Can you work these out from the drawing? Everything is in mm from the part's minimum corner. Give positions to 0.01 mm unless a question says otherwise; leave off trailing zeros. Write each loop counter-clockwise with the first axis right and the second up, starting at its lowest first coordinate (ties: lowest second). Pieces come first, ordered by that corner, then holes. Notation, with made-up numbers: M 89.5,-22.75 L 146.5,-22.75 A27 cw 146.5,-0.75 Z; hole C 66,83 d9. An arc over 180 degrees is marked long. One line per item, written item: value.
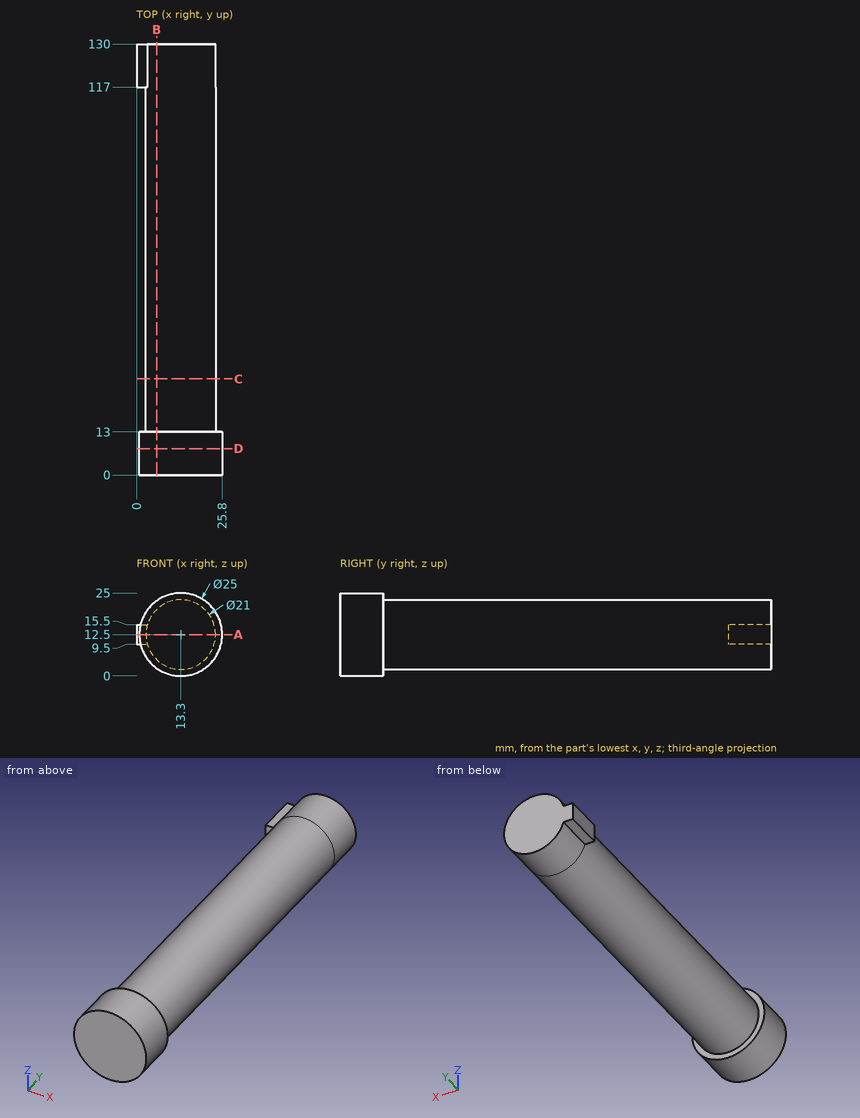
1) If we section it at D-D, the plane y = 8: Write out the boundary of the cut face in (x, z), then the cut area to 3 significant figures.
Outcome:
outline: C 13.3,12.5 d25
area: 491 mm^2
2) If we section it at B-B, the plane x = 6: Write out the boundary of the cut face in (y, z), then the cut area to 3 significant figures.
Outcome:
outline: M 0,2.35 L 13,2.35 L 13,4.95 L 130,4.95 L 130,20.05 L 13,20.05 L 13,22.65 L 0,22.65 Z
area: 2,030 mm^2
3) If we section it at C-C, the plane y = 29: Write out the boundary of the cut face in (x, z), then the cut area to 3 significant figures.
Outcome:
outline: C 13.3,12.5 d21
area: 346 mm^2
4) Please list where these lines run through material, in increasing order: L1, parallel to Y at x = 24.25, z = 14; L2, parallel to Z at x = 14, y = 18; L3, parallel to X at y = 120.5, z = 12.75. Write a range as from..to.
Outcome:
L1: y = 0..13
L2: z = 2.02..22.98
L3: x = 0..23.8
5) If we section it at A-A, the plane z = 12.5: Write out the boundary of the cut face in (x, y).
Outcome:
outline: M 0,117 L 2.8,117 L 2.8,13 L 0.8,13 L 0.8,0 L 25.8,0 L 25.8,13 L 23.8,13 L 23.8,130 L 0,130 Z
6) I'm going to push flat-ended pins straight in: pin 1 (2 mm diameter, centred on x = 20.5, y = 83.5, fed in from -Z) (1 decimal); pin 2 (3.5 mm diameter, centred on x = 2, y = 125, fed in from +Z) (1 decimal); pin 3 (5 mm diameter, centred on y = 68, z = 20.5, fed in from -X). Where does each tip first touch, or does it pass through?
Outcome:
pin 1: stops at z = 4
pin 2: stops at z = 16.9
pin 3: stops at x = 4.36
